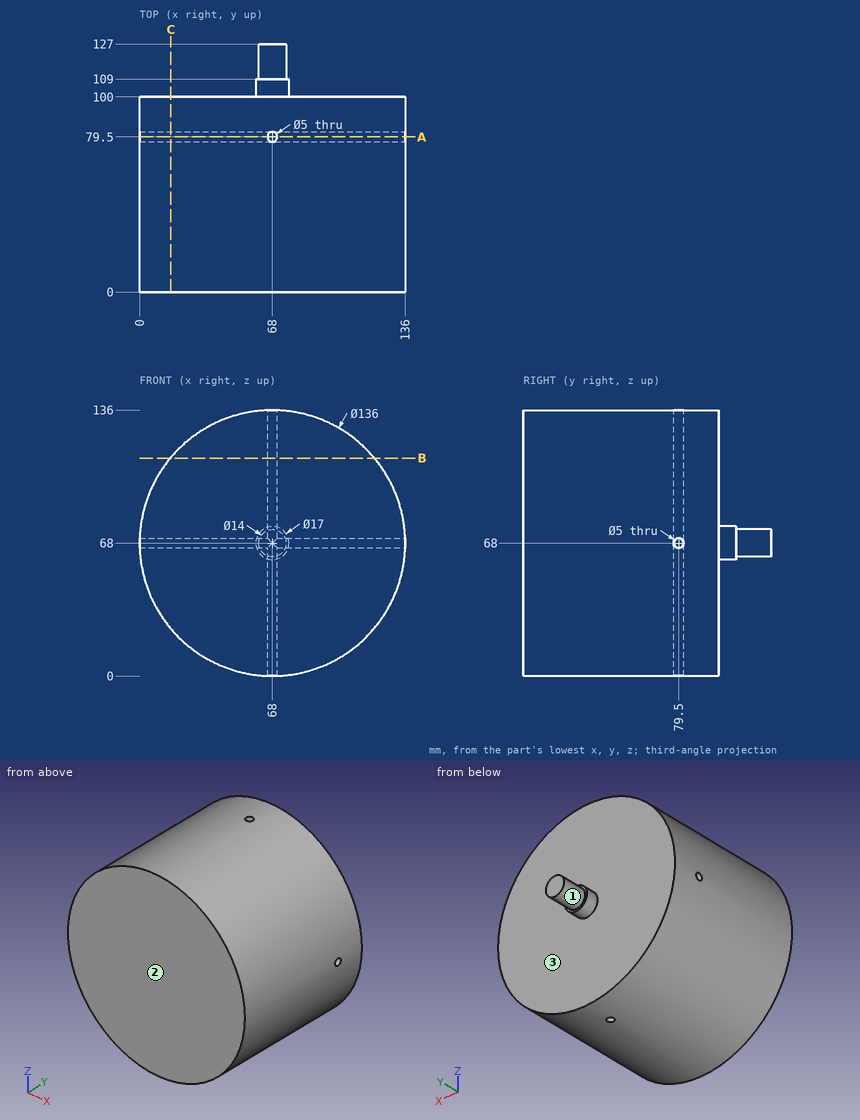
Could you check a few things on this drawing? It's one solid part, dimensions in mm from its lowest x, y, z. Coordinates: 2 decimals unless noted, no trailing zeros. Write each loop counter-clockwise with the first axis right and the second up, starting at its lowest first coordinate (ties: lowest second). Pieces come first, ordered by that corner, then holes. Notation, with made-up numbers: (-27, -12.75) - (-5, -12.75) arc R22 cw to (-5, 16.25) - close; hole circle Ø11 at (35, -15). An arc over 180 degrees is marked (long way). Write item = value, one per line.
1) We'd pull the mould along Y, two halves only. Please class the marked faces 1, 2 and 3: +Y half, -Y half, draft (parallel to the pull), parting line (faces both ways), or undercut.
Result set:
face_1 = draft
face_2 = -Y half
face_3 = +Y half
2) Will these pins go through, and if not, where does the flat tip stop? pin 1 Ø3 at (y, z) = (47.5, 102.5) entering from -X; pin 2 Ø4 at (x, y) = (49, 91) entering from +Z; pin 3 Ø8 at (x, y) = (31.5, 38.5) entering from -Z; pin 4 Ø4 at (y, z) = (79.5, 68) entering from +X.
Result set:
pin_1 = 8.54
pin_2 = 133.84
pin_3 = 8.27
pin_4 = through
3) Suppose I cut it at C-C on x = 16. Please give me the cut outline in (y, z).
Result set:
outline = (0, 24.18) - (100, 24.18) - (100, 111.82) - (0, 111.82) - close; hole circle Ø5 at (79.5, 68)
4) Please list where these lines run through material, in increasing order: line 1 (Z direction, x = 70, y = 63); line 2 (Y direction, x = 117.5, z = 34); line 3 (Y direction, x = 68, z = 30). Write a range as [from, to].
Result set:
line_1 = [0.03, 135.97]
line_2 = [0, 100]
line_3 = [0, 77], [82, 100]
5) Suppose I cut it at A-A on y = 79.5. Please give me the cut outline in (x, z).
Result set:
outline = (0.05, 65.5) arc R68 ccw to (65.5, 0.05) - (65.5, 65.5) - close; (0.05, 70.5) - (65.5, 70.5) - (65.5, 135.95) arc R68 ccw to start; (70.5, 0.05) arc R68 ccw to (135.95, 65.5) - (70.5, 65.5) - close; (70.5, 70.5) - (135.95, 70.5) arc R68 ccw to (70.5, 135.95) - close
6) Suppose I cut it at B-B on z = 111.5. Please give me the cut outline in (x, y), plus the area to 3 significant figures.
Result set:
outline = (15.73, 0) - (120.27, 0) - (120.27, 100) - (15.73, 100) - close; hole circle Ø5 at (68, 79.5)
area = 10,400 mm2
